```python
from build123d import *

# Parameters (mm, degrees)
CROQUIS2_R              = 40
CROQUIS2_R_2            = 37.5
SALIENTE_EXTRUIR1_DEPTH = 12
CROQUIS3_R              = 40
CROQUIS3_R_2            = 37.5
CROQUIS3_R_3            = 35
SALIENTE_EXTRUIR2_DEPTH = 3
CROQUIS4_R              = 40
SALIENTE_EXTRUIR3_DEPTH = 2.5


with BuildPart() as part:
    # Croquis2 → Saliente-Extruir1 (new body)
    with BuildSketch(Plane.XY.offset(34)):
        with Locations((13.541348433, 6.626768313)):
            Circle(CROQUIS2_R)
        with Locations((13.541348433, 6.626768313)):
            Circle(CROQUIS2_R_2, mode=Mode.SUBTRACT)
    extrude(amount=SALIENTE_EXTRUIR1_DEPTH)

    # Croquis3 → Saliente-Extruir2 (add)
    with BuildSketch(Plane.XY.offset(46)):
        with Locations((13.541348433, 6.626768313)):
            Circle(CROQUIS3_R)
        with Locations((13.541348433, 6.626768313)):
            Circle(CROQUIS3_R_2, mode=Mode.SUBTRACT)
        with Locations((13.541348433, 6.626768313)):
            Circle(CROQUIS3_R_3)
    extrude(amount=SALIENTE_EXTRUIR2_DEPTH)

    # Croquis4 → Saliente-Extruir3 (add)
    with BuildSketch(Plane.XY.offset(49)):
        with Locations((13.541348433, 6.626768313)):
            Circle(CROQUIS4_R)
    extrude(amount=SALIENTE_EXTRUIR3_DEPTH)


solid = part.part
```
Geometry: final body of the model. Coordinates: model frame, mm. A direction names the side the tool comes from. Coordinates: 2 decimals unless noted, no trailing zeros. Order: outer loops, then holes, each group sorted by start corner. A loop starts at its lowest first (then second) coordinate and runs counter-clockwise, first axis right, second up. Notation, with made-up numbers: M 13,-3 L 17,-3 A18 ccw 17,20 Z; hole C -14,36.25 d10. An arc over 180 degrees is marked long. Answer in a Markdown table with one row per item. Add a question column.
Q1. Reachability of faces 4 (the flat face through (13, 7, 51.5)), 5 (the flat face through (2, -27, 49)) from +Z, -Z, +X, -X, +Y, -Y: full face, straight path, thin tool, end or side. Return the list, or none.
Q2. Contact query for flat-ended pins moving along their axis: P1, Ø8, axis at x = -14.5, z = 43.5, coming from the +Y side; P2, Ø8, axis at x = 34, y = 22.5, coming from the -Z side; P3, Ø3, axis at x = 40, z = 40.5, coming from the -Y side. Output: stop coordinate, or through.
Q3. Section query B-B on x = 19.5. Return the cut outline in (y, z).
Q4. Line query: L1, parallel to Y at x = 19, z = 48.5; L2, parallel to Z at x = 11, y = 8.5; L3, parallel to Z at x = 38, y = -21. Output: solid intervals per line, ascending.
Q5. Mould query, pull axis X, two halves, no side actions, for faces 1 (the flat face through (13, 7, 46)), 2 (the flat face through (1.5, 42.4, 34)), 3 (the cylindrical face through (-18.201, -17.713, 42.628)). Classes: released by +X, released by -X, zero draft, split by the parting line, or undercut.
Q6. Section query A-A on y = 12. Return the cut outline in (x, z).
Q7. Section query C-C on z = 40.25. Return the cut outline in (x, y).
Completed:
| question | item | result |
|---|---|---|
| 1 | face 4 | +Z, +X, -X, +Y, -Y |
| 1 | face 5 | -Z |
| 2 | P1 | stops at y = 38.6 |
| 2 | P2 | stops at z = 46 |
| 2 | P3 | stops at y = -24.63 |
| 3 | outline | M -32.93,34 L -30.4,34 L -30.4,49 L -27.86,49 L -27.86,46 L 41.12,46 L 41.12,49 L 43.65,49 L 43.65,34 L 46.18,34 L 46.18,51.5 L -32.93,51.5 Z |
| 4 | L1 | y = -33 to -30.47, -27.94 to 41.2, 43.73 to 46.25 |
| 4 | L2 | z = 46 to 51.5 |
| 4 | L3 | z = 49 to 51.5 |
| 5 | face 1 | undercut |
| 5 | face 2 | zero draft |
| 5 | face 3 | split by the parting line |
| 6 | outline | M -26.1,34 L -23.57,34 L -23.57,49 L -21.04,49 L -21.04,46 L 48.13,46 L 48.13,49 L 50.65,49 L 50.65,34 L 53.18,34 L 53.18,51.5 L -26.1,51.5 Z |
| 7 | outline | C 13.54,6.63 d80; hole C 13.54,6.63 d75 |
